The listing builds one solid part. Answer for the finished solid, in the listing's coordinates (mm). Face numbers are marked on the shaded views. A direction names the side the tool comes from. Coordinates: 2 decimals unless noted, no trailing zeros. Loops run counter-clockwise (first coordinate to the right, second up) from the corner with the lowest first, then second, coordinate; pieces in that order, holes last. Notation, with made-up numbers: (47.25, 52) - (68.25, 52) arc R18 cw to (68.25, 74) - close; hole circle Ø2 at (-30, -10.75). An arc over 180 degrees is marked (long way). Return JSON: item names as keys, results as strings. Group by question number.
1. Section C-C (y = 5.5) is taken. Write down the section's boundary in (x, z), and give its area (3 significant figures).
2. Section D-D (x = -1.5) is taken. Write down the section's boundary in (y, z).
3. Each of these flat-tipped pins is pushed along its axis until it touches: P1, Ø2.5, axis at y = 7.5, z = 7.5, coming from the -X side; P2, Ø3, axis at x = -12, z = -11, coming from the +Y side; P3, Ø12, axis at x = -9, z = 1, coming from the -Y side. Where does it stop, or does it pass through?
4. Section B-B (z = -11.5) is taken. Write down the section's boundary in (x, y).
5. The mould has two halves that part along X. Classify the marked faces 4, 5 and 6: pulls with the +X half, pulls with the -X half, needs draft (parallel to the pull), parting line crosses it, or undercut.
6. Find the intervals of material crossed by line 1 along X through (y, z) = (7, -12); line 2 along Z through (x, y) = (8.5, 7); line 3 along X through (y, z) = (1.75, -18), in increasing order.
7. Section A-A (x = -12.9) is taken. Write down the section's boundary in (y, z).
8. Which of the six approach directions +Z, -Z, +X, -X, +Y, -Y give full straight-line access (tool end or side, diameter ignored) to the marked faces 1, 2 and 3?
Autodesk Inventor part; units mm, degrees
ref_plane "YZ Plane" through (0, 0, 0) normal (1, 0, 0) x (0, 1, 0)
ref_plane "XZ Plane" through (0, 0, 0) normal (0, 1, 0) x (-1, 0, 0)
ref_plane "XY Plane" through (0, 0, 0) normal (0, 0, 1) x (1, 0, 0)
sketch "Sketch1" plane through (0, 0, 0) normal (0, 1, 0) x (-1, 0, 0)
  line L0 (8.9, 21.65) -> (-8.9, 21.65)
  line L1 (-8.9, 21.65) -> (-8.9, -21.65)
  line L2 (-8.9, -21.65) -> (8.9, -21.65)
  line L3 (8.9, -21.65) -> (8.9, 21.65)
  line L4 (8.9, 21.65) -> (-8.9, -21.65) construction
  line L5 (-8.9, 21.65) -> (8.9, -21.65) construction
  line L6 (9.9, 22.65) -> (-9.9, 22.65)
  line L7 (-9.9, 22.65) -> (-9.9, -22.65)
  line L8 (-9.9, -22.65) -> (9.9, -22.65)
  line L9 (9.9, -22.65) -> (9.9, 22.65)
  line L10 (9.9, 22.65) -> (-9.9, -22.65) construction
  line L11 (-9.9, 22.65) -> (9.9, -22.65) construction
  line L12 (9.9, 22.65) -> (15.9, 22.65)
  line L13 (15.9, 22.65) -> (15.9, -22.65)
  line L14 (15.9, -22.65) -> (9.9, -22.65)
  line L15 (9.9, -22.65) -> (9.9, 22.65)
  line L16 (8.9, -21.65) -> (8.9, -22.65)
  line L17 (-8.9, -21.65) -> (-8.9, -22.65)
  line L18 (12.9, 19.85) -> (12.9, -20.15) construction
  line L19 (11.25, 19.85) -> (11.25, -20.15)
  line L20 (14.55, -20.15) -> (14.55, 19.85)
  arc A0 (14.55, 19.85) -> (11.25, 19.85) centre (12.9, 19.85) ccw
  arc A1 (11.25, -20.15) -> (14.55, -20.15) centre (12.9, -20.15) ccw
  point P0 (0, 0)
  point P1 (12.9, -0.15)
  point P2 (12.9, -22.65)
  dimension "d0" = 17.8
  dimension "d1" = 43.3
  dimension "d2" = 19.8
  dimension "d3" = 45.3
  dimension "d4" = 6
  dimension "d5" = 3.3
  dimension "d6" = 40
  dimension "d7" = 2.5
extrude "Extrusion1" add sketch "Sketch1" along normal blind 2 contours L3 L2 L1 L0 | L16 L8 L17 L2 | L9 L12 L13 L14
extrude "Extrusion2" add sketch "Sketch1" along normal blind 10 contours L0 L1 L17 L8 L7 L6 L9 L16 L3
properties part number "Mounting Relay"
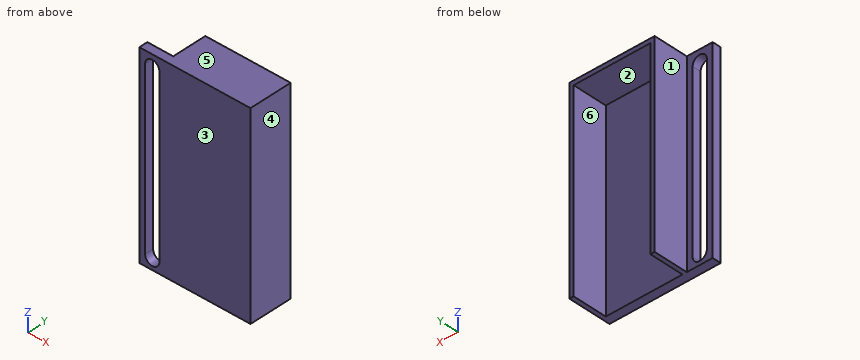
The answers:
{
 "1": {"outline": "(-9.9, -22.65) - (-8.9, -22.65) - (-8.9, 21.65) - (8.9, 21.65) - (8.9, -22.65) - (9.9, -22.65) - (9.9, 22.65) - (-9.9, 22.65) - close", "area": "108 mm2"},
 "2": {"outline": "(0, -22.65) - (2, -22.65) - (2, 21.65) - (10, 21.65) - (10, 22.65) - (0, 22.65) - close"},
 "3": {"P1": "stops at x = -9.9", "P2": "stops at y = 2", "P3": "stops at y = 0"},
 "4": {"outline": "(-15.9, 0) - (-14.55, 0) - (-14.55, 2) - (-15.9, 2) - close; (-11.25, 0) - (9.9, 0) - (9.9, 10) - (8.9, 10) - (8.9, 2) - (-8.9, 2) - (-8.9, 10) - (-9.9, 10) - (-9.9, 2) - (-11.25, 2) - close"},
 "5": {"face 4": "pulls with the +X half", "face 5": "needs draft", "face 6": "undercut"},
 "6": {"line 1": "x = -9.9 to -8.9, 8.9 to 9.9", "line 2": "z = 21.65 to 22.65", "line 3": "x = -15.9 to -14.55, -11.25 to 9.9"},
 "7": {"outline": "(0, -22.65) - (2, -22.65) - (2, -21.8) - (0, -21.8) - close; (0, 21.5) - (2, 21.5) - (2, 22.65) - (0, 22.65) - close"},
 "8": {"face 1": "+Z, -Z, -X, +Y", "face 2": "-Z, +Y", "face 3": "+Z, -Z, +X, -X, -Y"}
}
